Here's how the part is built. I have some questions about the finished solid (model axes, mm). A direction names the side the tool comes from. Round coordinates to 2 decimals unless told otherwise and drop trailing zeros. Order: outer loops, then holes, each group sorted by start corner. A loop starts at its lowest first (then second) coordinate and runs counter-clockwise, first axis right, second up.
Autodesk Fusion 360 part; units mm, degrees
sketch "Schizzo1" plane through (0, 0, 0) normal (0, 0, 1) x (1, 0, 0)
  circle A0 centre (10.2944, 3.2873) radius 1.4
  circle A1 centre (10.2944, 3.2873) radius 3.3
  line L0 (13.5944, 3.0373) -> (6.9944, 3.0373)
  line L1 (6.9944, 3.0373) -> (6.9944, 3.5373)
  line L2 (6.9944, 3.5373) -> (13.5944, 3.5373)
  line L3 (13.5944, 3.5373) -> (13.5944, 3.0373)
  line L4 (13.5944, 3.0373) -> (6.9944, 3.5373) construction
  line L5 (6.9944, 3.0373) -> (13.5944, 3.5373) construction
  line L6 (10.5444, -0.0127) -> (10.0444, -0.0127)
  line L7 (10.0444, -0.0127) -> (10.0444, 6.5873)
  line L8 (10.0444, 6.5873) -> (10.5444, 6.5873)
  line L9 (10.5444, 6.5873) -> (10.5444, -0.0127)
  line L10 (10.5444, -0.0127) -> (10.0444, 6.5873) construction
  line L11 (10.0444, -0.0127) -> (10.5444, 6.5873) construction
  circle A2 centre (10.2944, 3.2873) radius 1.5
  point P0 (10.2944, 3.2873)
  point P1 (10.2944, 3.2873)
  dimension "d1" = 2.8
  dimension "d2" = 6.6
  dimension "d3" = 0.5
  dimension "d4" = 0.5
  dimension "d16" = 3
extrude "Estrusione1" add sketch "Schizzo1" along normal blind 9 contours A0 L2 L9 A2 | A0 L0 L9 A2 | A1 L2 L9 A2 | A1 L0 L9 A2 | A0 L2 L7 A2 | A0 L0 L7 A2 | A1 L2 L7 A2 | A1 L0 L7 A2 makes body 1 at (7.1541, 4.3014, 6) makes body 2 at (7.5637, 1.4344, 6) makes body 3 at (12.397, 5.8308, 6) makes body 4 at (13.3249, 1.9811, 6)
extrude "Estrusione2" add sketch "Schizzo1" along normal blind 1 from surface at 9 contours A1 L2 L9 A2 | A1 L0 L2 A2 | A1 L0 L9 A2 | A1 L7 L9 A2 | A1 L7 L9 A2 | A1 L2 L7 A2 | A1 L0 L7 A2 | A1 L0 L2 A2 bodies 1 2 3 4
sketch "Schizzo2" plane through (0, 0, 10) normal (0, 0, 1) x (-1, 0, 0)
  circle A0 centre (-10.2944, -3.2873) radius 3.3
  line L0 (-14.2944, 0.7127) -> (-6.2944, 0.7127)
  line L1 (-6.2944, 0.7127) -> (-6.2944, -7.2873)
  line L2 (-6.2944, -7.2873) -> (-14.2944, -7.2873)
  line L3 (-14.2944, -7.2873) -> (-14.2944, 0.7127)
  line L4 (-14.2944, 0.7127) -> (-6.2944, -7.2873) construction
  line L5 (-6.2944, 0.7127) -> (-14.2944, -7.2873) construction
  circle A1 centre (-10.2944, -3.2873) radius 3
  circle A2 centre (-10.2944, -3.2873) radius 1.5
  point P0 (-10.2944, -3.2873)
  dimension "d10" = 8
  dimension "d11" = 8
  dimension "d13" = 6
extrude "Estrusione3" add sketch "Schizzo2" along normal blind 3 contours A0 | L0 L1 L2 L3 bodies 1
extrude "Estrusione4" add sketch "Schizzo2" along normal blind 1 contours A1 bodies 1
1. If we section it at B-B, the plane x = 9.5: Write out the boundary of the cut face in (y, z), and give its area (3 significant figures).
Evaluation:
outline: (-0.71, 10) - (0.08, 10) - (0.08, 0) - (2.13, 0) - (2.13, 9) - (2.01, 9) - (2.01, 11) - (0.39, 11) - (0.39, 13) - (-0.71, 13) - close; (4.44, 0) - (6.49, 0) - (6.49, 10) - (7.29, 10) - (7.29, 13) - (6.18, 13) - (6.18, 11) - (4.56, 11) - (4.56, 9) - (4.44, 9) - close
area: 50.6 mm2
2. If we section it at C-C, the plane y = 2.75: Write out the boundary of the cut face in (x, z), and give its area (3 significant figures).
Evaluation:
outline: (6.29, 10) - (7.04, 10) - (7.04, 0) - (9, 0) - (9, 9) - (8.89, 9) - (8.89, 11) - (7.34, 11) - (7.34, 13) - (6.29, 13) - close; (11.59, 0) - (13.55, 0) - (13.55, 10) - (14.29, 10) - (14.29, 13) - (13.25, 13) - (13.25, 11) - (11.69, 11) - (11.69, 9) - (11.59, 9) - close
area: 48.4 mm2
3. If we section it at D-D, the plane x = 12.25: Write out the boundary of the cut face in (y, z).
Evaluation:
outline: (-0.71, 10) - (0.63, 10) - (0.63, 0) - (3.04, 0) - (3.04, 9) - (3.54, 9) - (3.54, 0) - (5.95, 0) - (5.95, 10) - (7.29, 10) - (7.29, 13) - (5.56, 13) - (5.56, 11) - (1.01, 11) - (1.01, 13) - (-0.71, 13) - close
4. If we section it at A-A, the plane z = 5.25: Write out the boundary of the cut face in (x, y), and give its area (3 significant figures).
Evaluation:
outline: (7, 3.04) arc R3.3 ccw to (10.04, 0) - (10.04, 1.91) arc R1.4 cw to (8.92, 3.04) - close; (7, 3.54) - (8.92, 3.54) arc R1.4 cw to (10.04, 4.66) - (10.04, 6.58) arc R3.3 ccw to start; (10.54, 0) arc R3.3 ccw to (13.58, 3.04) - (11.67, 3.04) arc R1.4 cw to (10.54, 1.91) - close; (10.54, 4.66) arc R1.4 cw to (11.67, 3.54) - (13.58, 3.54) arc R3.3 ccw to (10.54, 6.58) - close
area: 24.2 mm2
5. I'm going to push flat-ended pins straight in: P1, Ø0.6, axis at x = 9.5, y = 4, coming from the +Z side; P2, Ø3, axis at x = 10, y = 4, coming from the +Z side; P3, Ø1.5, axis at x = 13, z = 5, coming from the +Y side; P4, Ø2, axis at x = 8.5, z = 4, coming from the +Y side. Where does each tip first touch, or does it pass through?
Evaluation:
P1: passes through
P2: stops at z = 11
P3: stops at y = 5.95
P4: stops at y = 6.49
6. On a 3-axis mill with a long thin cutter (end or side, diameter ignored), from which of +Z, -Z, +X, -X, +Y, -Y can I reach the whole of each face in a straight line? I mean faces 1 (the flat face through (10.544, 6, 4)), 2 (the flat face through (8, 3.037, 4)), 3 (the cylindrical face through (11.293, 2.306, 4.437)), 4 (the cylindrical face through (12.675, 1.462, 11.986)), 5 (the flat face through (14, 3, 10)). Say none if no direction works.
Evaluation:
face 1: -Z, +Y, -Y
face 2: -Z, +X, -X
face 3: +Z, -Z
face 4: +Z
face 5: -Z
7. I need wall thicknesses on probe 1 along X at (y, z) = (3.75, 7.25); probe 2 along Z at (x, y) = (12.5, 1.75); probe 3 along Z at (x, y) = (13.75, -0.25). Which ranges of each line are inside material? Lowest first, please.
Evaluation:
probe 1: x = 7.03 to 8.97, 11.62 to 13.56
probe 2: z = 0 to 11
probe 3: z = 10 to 13
8. If we mould it in two halves opening along X, with no side actions, what happens to faces 6 (the cylindrical face through (11.276, 4.286, 4.437)), 7 (the flat face through (12, 5, 0))? For each: released by +X, released by -X, zero draft, split by the parting line, or undercut.
Evaluation:
face 6: undercut
face 7: zero draft
